Design review of the part built by this model. Coordinates are the model's own, in mm. A direction names the side the tool comes from. Round coordinates to 2 decimals unless told otherwise and drop trailing zeros. Order: outer loops, then holes, each group sorted by start corner. A loop starts at its lowest first (then second) coordinate and runs counter-clockwise, first axis right, second up. Notation, with made-up numbers: M 37,-16 L 43,-16 A20 cw 43,-2 Z; hole C 34,28.5 d10. An arc over 180 degrees is marked long. Write item = value, one per line. Start each with the question number.
```python
from build123d import *

# Parameters (mm, degrees)
PAD_DEPTH       = 9.75
SKETCH001_R     = 1.6
POCKET_DEPTH    = 9.751
SKETCH002_R     = 1.6
POCKET001_DEPTH = 12.001
POCKET002_DEPTH = 2.4


with BuildPart() as part:
    # Sketch → Pad (new body)
    with BuildSketch(Plane.XY):
        with BuildLine():
            ThreePointArc((6, 7.5), (0, 13.5), (-6, 7.5))
            Line((-6, 7.5), (-6, -7.5))
            Line((-6, -7.5), (6, -7.5))
            Line((6, -7.5), (6, 7.5))
        make_face()
    extrude(amount=PAD_DEPTH)

    # Sketch001 (on Face5 of Pad) → Pocket (cut, through all)
    with BuildSketch(Plane(origin=(0, 0, 0), x_dir=(1, 0, 0), z_dir=(0, 0, -1))):
        with Locations((0, -7.5)):
            Circle(SKETCH001_R)
    extrude(amount=-POCKET_DEPTH, mode=Mode.SUBTRACT)

    # Sketch002 (on Face3 of Pocket) → Pocket001 (cut, through all)
    with BuildSketch(Plane(origin=(-6, 0, 0), x_dir=(0, -1, 0), z_dir=(-1, 0, 0))):
        with Locations((3, 4.875)):
            Circle(SKETCH002_R)
    extrude(amount=-POCKET001_DEPTH, mode=Mode.SUBTRACT)

    # Sketch003 (on Face3 of Pocket001) → Pocket002 (cut)
    with BuildSketch(Plane(origin=(-6, 0, 0), x_dir=(0, -1, 0), z_dir=(-1, 0, 0))):
        Polygon((5.8, 6.491581), (3, 8.108162), (0.2, 6.491581), (0.2, 3.258419), (3, 1.641838), (5.8, 3.258419), align=None)
    extrude(amount=-POCKET002_DEPTH, mode=Mode.SUBTRACT)


solid = part.part
```
(1) For line 1 along Z through (x, y) = (4, -3) (3 decimals); line 2 along Y through (x, z) = (0, 4); line 3 along Y through (x, z) = (0.5, 4), list the stretches that pass through material, from the lowest coordinate up. Write a range as [from, to].
(2) Consider section C-C, the plane z = 0.75. Write out the cut boundary in (x, y), then the cut area to 3 significant figures.
(3) Consider section A-A, the plane x = 0. Write out the cut boundary in (y, z) (3 decimals).
(4) For faces 5 (the face through (-6, 0, 5)), 6 (the face through (-4.82, -4.38, 2.44)), list the 3-axis set-ups (+Z, -Z, +X, -X, +Y, -Y) from which the entire face can be reached by the end or side of a thin tool; tool diameter is ignored.
(5) Insertion check: pin 1 (4 mm diameter, centred on y = 11, z = 2.5, fed in from +X); pin 2 (1.9 mm diameter, centred on x = -4.5, z = 5.5, fed in from +Y); pin 3 (1.7 mm diameter, centred on y = -3, z = 5, fed in from -X). Each pin has a flat end and moves straight along its axis. Give the tip position at first contact, or say it passes through.
(6) Consider section B-B, the plane y = 8. Write out the cut boundary in (x, z), then the cut area to 3 significant figures.
(7) Draft analysis for pull direction Z (two halves, no side actions). For faces 1 (the face through (6, 0, 5)), 2 (the face through (-4.8, -1.6, 7.3)), 3 (the face through (0, 3, 0)), 4 (the face through (0, 3, 9.75)), state which applies: pulls with the +Z half, pulls with the -Z half, needs draft (parallel to the pull), parting line crosses it, or undercut.
(8) Consider section D-D, the plane x = -2.5. Write out the cut boundary in (y, z) (3 decimals).
Completed:
q1.line_1 = [0, 3.275], [6.475, 9.75]
q1.line_2 = [-7.5, -4.34], [-1.66, 5.9], [9.1, 13.5]
q1.line_3 = [-7.5, -4.34], [-1.66, 5.98], [9.02, 13.48]
q2.outline = M -6,-7.5 L 6,-7.5 L 6,7.5 A6 ccw -6,7.5 Z; hole C 0,7.5 d3.2
q2.area = 229 mm2
q3.outline = M -7.5,0 L 5.9,0 L 5.9,9.75 L -7.5,9.75 Z; M 9.1,0 L 13.5,0 L 13.5,9.75 L 9.1,9.75 Z; hole C -3,4.875 d3.2
q4.face_5 = +Z, -Z, -X, +Y, -Y
q4.face_6 = -X
q5.pin_1 = 5.81
q5.pin_2 = 12.34
q5.pin_3 = through
q6.outline = M -5.98,0 L -1.52,0 L -1.52,9.75 L -5.98,9.75 Z; M 1.52,0 L 5.98,0 L 5.98,9.75 L 1.52,9.75 Z
q6.area = 87.0 mm2
q7.face_1 = needs draft
q7.face_2 = undercut
q7.face_3 = pulls with the -Z half
q7.face_4 = pulls with the +Z half
q8.outline = M -7.5,0 L 12.954,0 L 12.954,9.75 L -7.5,9.75 Z; hole C -3,4.875 d3.2
